from build123d import *

# Parameters (mm, degrees)
BOSS_EXTRUDE1_DEPTH = 304.8
FILLET1_R           = 3.175
SKETCH2_R           = 2.25
CUT_EXTRUDE1_DEPTH  = 4.175
SKETCH2_3_R         = 2.25
CUT_EXTRUDE2_DEPTH  = 4.175
SKETCH3_R           = 2.25
CUT_EXTRUDE3_DEPTH  = 4.175


with BuildPart() as part:
    # Sketch1 → Boss-Extrude1 (new body, symmetric)
    with BuildSketch(Plane.XY):
        Polygon((0, 25.4), (0, 0), (25.4, 0), (25.4, 3.175), (3.175, 3.175), (3.175, 25.4), align=None)
    extrude(amount=BOSS_EXTRUDE1_DEPTH, both=True)

    # Fillet1
    fillet1_edges = [part.edges().sort_by_distance(p)[0] for p in [
        (3.175, 3.175, 0),
    ]]
    fillet(fillet1_edges, radius=FILLET1_R)

    # Sketch2 → Cut-Extrude1 (cut, through all)
    with BuildSketch(Plane(origin=(0, 3.175, 0), x_dir=(1, 0, 0), z_dir=(0, 1, 0))):
        with Locations((13.758333333, -292.1)):
            Circle(SKETCH2_R)
        with Locations((22.225, -285.75)):
            Circle(SKETCH2_R)
        with Locations((13.758333333, 292.1)):
            Circle(SKETCH2_R)
        with Locations((22.225, 285.75)):
            Circle(SKETCH2_R)
    extrude(amount=-CUT_EXTRUDE1_DEPTH, mode=Mode.SUBTRACT)

    # Sketch2_3 → Cut-Extrude2 (cut, through all)
    with BuildSketch(Plane(origin=(0, 3.175, 0), x_dir=(1, 0, 0), z_dir=(0, 1, 0))):
        with Locations((19.05, -266.7)):
            Circle(SKETCH2_3_R)
        with Locations((19.05, -228.6)):
            Circle(SKETCH2_3_R)
        with Locations((19.05, -190.5)):
            Circle(SKETCH2_3_R)
        with Locations((19.05, -152.4)):
            Circle(SKETCH2_3_R)
        with Locations((19.05, -114.3)):
            Circle(SKETCH2_3_R)
        with Locations((19.05, -76.2)):
            Circle(SKETCH2_3_R)
        with Locations((19.05, -38.1)):
            Circle(SKETCH2_3_R)
        with Locations((19.05, 0)):
            Circle(SKETCH2_3_R)
        with Locations((19.05, 38.1)):
            Circle(SKETCH2_3_R)
        with Locations((19.05, 76.2)):
            Circle(SKETCH2_3_R)
        with Locations((19.05, 114.3)):
            Circle(SKETCH2_3_R)
        with Locations((19.05, 152.4)):
            Circle(SKETCH2_3_R)
        with Locations((19.05, 190.5)):
            Circle(SKETCH2_3_R)
        with Locations((19.05, 228.6)):
            Circle(SKETCH2_3_R)
        with Locations((19.05, 266.7)):
            Circle(SKETCH2_3_R)
    cut_extrude2 = extrude(amount=-CUT_EXTRUDE2_DEPTH, mode=Mode.SUBTRACT)

    # Mirror1: Cut-Extrude2 across plane
    add(cut_extrude2.mirror(Plane(origin=(0, 0, 0), x_dir=(0, 0, 1), z_dir=(-0.707106781, 0.707106781, 0))), mode=Mode.SUBTRACT)

    # Sketch3 → Cut-Extrude3 (cut, through all)
    with BuildSketch(Plane(origin=(3.175, 0, 0), x_dir=(0, 0, -1), z_dir=(1, 0, 0))):
        with Locations((-282.575, 22.225)):
            Circle(SKETCH3_R)
        with Locations((-291.041666667, 15.875)):
            Circle(SKETCH3_R)
        with Locations((291.041666667, 15.875)):
            Circle(SKETCH3_R)
        with Locations((282.575, 22.225)):
            Circle(SKETCH3_R)
    extrude(amount=-CUT_EXTRUDE3_DEPTH, mode=Mode.SUBTRACT)


solid = part.part
Source: CAD feature listing. Evaluate the final solid. Frame: model axes, mm. A direction names the side the tool comes from. Round coordinates to 2 decimals unless told otherwise and drop trailing zeros. Use a Markdown table: item, result. Add a question column.
1. Line query: probe 1 along Y at (x, z) = (1.7, -266.7); probe 2 along X at (y, z) = (20.25, 84.5) (3 decimals). Output: solid intervals per line, ascending.
2. Set-up query: faces 1 (the flat face through (13, 0, 4)), 2 (the flat face through (16, 3.175, 4)). Return all of +Z, -Z, +X, -X, +Y, -Y with unobstructed straight access to the full face (end or side cutting, diameter ignored); none if empty.
3. First-contact query: pin 1 (7 mm diameter, centred on y = 22.225, z = -282.575, fed in from +X) (3 decimals); pin 2 (3.5 mm diameter, centred on y = 19.05, z = -266.7, fed in from +X); pin 3 (1 mm diameter, centred on y = 4.5, z = 186.5, fed in from +X) (3 decimals); pin 4 (7 mm diameter, centred on x = 22.225, z = -285.75, fed in from +Y) (3 decimals). Flat tips, straight axial feed; report the tip coordinate or a pass-through.
Derived:
| question | item | result |
|---|---|---|
| 1 | probe 1 | 0 to 16.8, 21.3 to 25.4 |
| 1 | probe 2 | 0 to 3.175 |
| 2 | face 1 | +Z, -Z, +X, -X, -Y |
| 2 | face 2 | +Z, -Z, +X, +Y |
| 3 | pin 1 | x = 3.175 |
| 3 | pin 2 | through |
| 3 | pin 3 | x = 4.215 |
| 3 | pin 4 | y = 3.175 |
